Read the model definition and answer for the solid it produces. Units are mm, in the model's axes. A direction names the side the tool comes from. Give positions to 0.01 mm unless a question says otherwise; leave off trailing zeros. Write each loop counter-clockwise with the first axis right and the second up, starting at its lowest first coordinate (ties: lowest second). Pieces come first, ordered by that corner, then holes.
```python
from build123d import *

# Parameters (mm, degrees)
SWEEP_THIN1_PROFILE_R   = 145
SWEEP_THIN1_PROFILE_R_2 = 105


with BuildPart() as part:
    # Sweep-Thin1: sweep along a path in Sketch1
    with BuildLine(Plane.XY) as sweep_thin1_path:
        Line((0, 0), (-150, 0))
        ThreePointArc((-150, 0), (-333.847763109, 76.152236891), (-410, 260))
        Line((-410, 260), (-410, 410))
    # Sweep-Thin1 profile (on start of the path) → Sweep-Thin1 (sweep)
    with BuildSketch(Plane(origin=(0, 0, 0), x_dir=(0, -1, 0), z_dir=(-1, 0, 0))):
        Circle(SWEEP_THIN1_PROFILE_R)
        Circle(SWEEP_THIN1_PROFILE_R_2, mode=Mode.SUBTRACT)
    sweep(path=sweep_thin1_path.line)


solid = part.part
```
Item 1: Determine the mould class of faces 1 (the cylindrical face through (-305.1, 336, 4.6)), 2 (the cylindrical face through (-76.05, -100.15, 31.54)), 3 (the cylindrical face through (-548.304, 336.05, 43.554)) for opening direction X: pulls with the +X half, pulls with the -X half, needs draft (parallel to the pull), parting line crosses it, or undercut.
Result set:
face 1: undercut
face 2: needs draft
face 3: parting line crosses it
Item 2: Section D-D (z = 122.5) is taken. Write down the section's boundary in (x, y).
Result set:
outline: (-487.58, 260) arc R337.58 ccw to (-150, -77.58) - (0, -77.58) - (0, 77.58) - (-150, 77.58) arc R182.42 cw to (-332.42, 260) - (-332.42, 410) - (-487.58, 410) - close
Item 3: Find the intervals of material crossed by line 1 along Z through (x, y) = (-78, 0); line 2 along Y through (x, z) = (-316.5, 81.5); line 3 along Z through (x, y) = (-391, 138.5), in increasing order.
Result set:
line 1: z = -145 to -105, 105 to 145
line 2: y = -81.5 to -20.51, 160.83 to 410
line 3: z = -144.66 to -104.53, 104.53 to 144.66
Item 4: Section B-B (x = -69) is taken. Write down the section's boundary in (y, z), and give its area (3 significant figures).
Result set:
outline: circle Ø290 at (0, 0); hole circle Ø210 at (0, 0)
area: 31,400 mm2
Item 5: Which of the six approach directions +Z, -Z, +X, -X, +Y, -Y give full straight-line access (tool end or side, diameter ignored) to faces 4 (the cylindrical face through (-76.05, -138.304, 43.554)), 5 (the flat face through (0, -44, -96))?
Result set:
face 4: +X
face 5: +Z, -Z, +X, +Y, -Y
Item 6: Section A-A (z = 0) is taken. Write down the section's boundary in (x, y).
Result set:
outline: (-555, 260) arc R405 ccw to (-150, -145) - (0, -145) - (0, -105) - (-150, -105) arc R365 cw to (-515, 260) - (-515, 410) - (-555, 410) - close; (-305, 260) arc R155 ccw to (-150, 105) - (0, 105) - (0, 145) - (-150, 145) arc R115 cw to (-265, 260) - (-265, 410) - (-305, 410) - close
Item 7: Section C-C (z = -86.5) is taken. Write down the section's boundary in (x, y), and give its area (3 significant figures).
Result set:
outline: (-526.37, 260) arc R376.37 ccw to (-150, -116.37) - (0, -116.37) - (0, -59.52) - (-150, -59.52) arc R319.52 cw to (-469.52, 260) - (-469.52, 410) - (-526.37, 410) - close; (-350.48, 260) arc R200.48 ccw to (-150, 59.52) - (0, 59.52) - (0, 116.37) - (-150, 116.37) arc R143.63 cw to (-293.63, 260) - (-293.63, 410) - (-350.48, 410) - close
area: 80,500 mm2
Item 8: Each of these flat-tipped pins is pushed along its axis until it touches: pin 1 Ø1.5 at (x, z) = (-191, -40.5) entering from -Y; pin 2 Ø8 at (y, z) = (-60.5, -56.5) entering from -X; pin 3 Ø8 at (x, y) = (-116.5, -12.5) entering from +Z. Where does it stop, or does it pass through?
Result set:
pin 1: stops at y = -137.35
pin 2: stops at x = -384.56
pin 3: stops at z = 144.75
